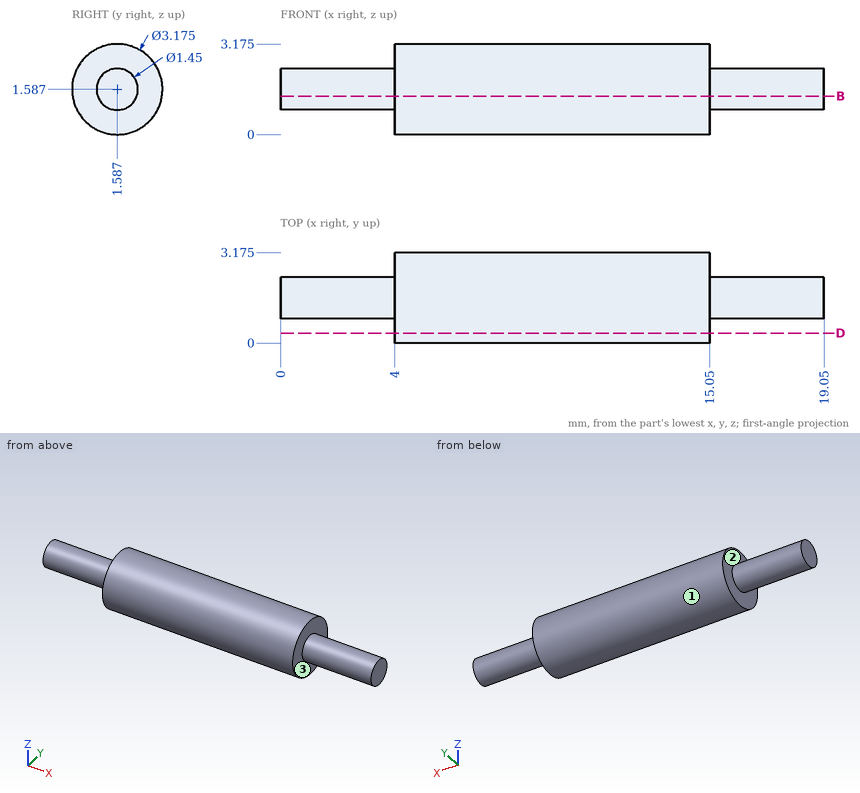
Here's the drawing with two shaded views (mm, measured from the low corner). I have some questions. A direction names the side the tool comes from. Round coordinates to 2 decimals unless told otherwise and drop trailing zeros. Write each loop counter-clockwise with the first axis right and the second up, starting at its lowest first coordinate (ties: lowest second). Pieces come first, ordered by that corner, then holes. Notation, with made-up numbers: M 47,-10 L 68,-10 A20 ccw 68,17 Z; hole C 72.25,-26 d10. An arc over 180 degrees is marked long. Use CSV: the item, a comma, the result in double quotes.
(1) I need wall thicknesses on line 1 along X through (y, z) = (0.75, 2.7); line 2 along Y through (x, z) = (10.5, 1.7) (1 decimal); line 3 along Z through (x, y) = (13.25, 0.3) (1 decimal). Which ranges of each line are inside material? Lowest first, please.
Check values:
line 1,"4 to 15.05"
line 2,"0 to 3.2"
line 3,"0.7 to 2.5"
(2) I'm going to push a flat-ended pin straight in: pin 1 (1 mm diameter, centred on x = 14.5, z = 2.5, fed in from -Y) (1 decimal). Where does the tip first touch, or does it pass through?
Check values:
pin 1,"y = 0.1"
(3) Imagine slicing it at D-D (y = 0.35). Write out the boundary of the cut face in (x, z).
Check values:
outline,"M 4,0.59 L 15.05,0.59 L 15.05,2.58 L 4,2.58 Z"
(4) Imagine slicing it at B-B (z = 1.35). Write out the boundary of the cut face in (x, y).
Check values:
outline,"M 0,0.9 L 4,0.9 L 4,0.02 L 15.05,0.02 L 15.05,0.9 L 19.05,0.9 L 19.05,2.27 L 15.05,2.27 L 15.05,3.16 L 4,3.16 L 4,2.27 L 0,2.27 Z"
(5) On a 3-axis mill with a long thin cutter (end or side, diameter ignored), from which of +Z, -Z, +X, -X, +Y, -Y can I reach the whole of each face in a straight line? I mean the marked faces 1, 2 and 3. Say none if no direction works.
Check values:
face 1,"+X, -X"
face 2,"-X"
face 3,"+X"
